Here's how the part is built. I have some questions about the finished solid (model axes, mm). A direction names the side the tool comes from. Give positions to 0.01 mm unless a question says otherwise; leave off trailing zeros. Order: outer loops, then holes, each group sorted by start corner. A loop starts at its lowest first (then second) coordinate and runs counter-clockwise, first axis right, second up. Notation, with made-up numbers: (21.5, 71.5) -> (32.5, 71.5) arc R20 cw to (32.5, 90.5) -> close; hole circle Ø10 at (-34, 8.25). An arc over 180 degrees is marked (long way). Write each question's results on one line, items separated by ' | '. Start each with the question number.
Q1. Imagine slicing it at D-D, the plane z = -16.5. Please give me the cut outline in (x, y), then the cut area to 3 significant figures.
Q2. Thinking about a two-plate mould opening in Z: for faces 1 (the face through (3.13, 28.27, -28.19)), 2 (the face through (3, 0, -26)), 3 (the face through (3.131, 1.528, -1.449)), which applies, pulls with the +Z half, pulls with the -Z half, needs draft (parallel to the pull), parting line crosses it, or undercut?
Q3. Imagine slicing it at A-A, the plane y = 51.5. Please give me the cut outline in (x, z).
Q4. Imagine slicing it at B-B, the plane z = -23. Please give me the cut outline in (x, y).
Q5. I need wall thicknesses on line 1 along Z through (x, y) = (4.75, 51); line 2 along Y through (x, z) = (5, -22); line 3 along Y through (x, z) = (1, -19). Which ranges of each line are inside material? Lowest first, please. Write a range as [from, to].
Q6. I'm going to push flat-ended pins straight in: pin 1 (1.9 mm diameter, centred on x = 4.5, y = 17.5, fed in from +Z); pin 2 (1.9 mm diameter, centred on x = 1.5, y = 2.5, fed in from +Z). Where does each tip first touch, or does it pass through?
Q7. For faces 4 (the face through (3, 29.718, -13)), 5 (the face through (3, 49, -29.718)), 6 (the face through (3, 33, -14.859)), which set-ups out of +Z, -Z, +X, -X, +Y, -Y let a thin tool reach every point of the face, with its end or its side?
Q8. Imagine slicing it at C-C, the plane x = 1. Please give me the cut outline in (y, z).
```python
from build123d import *

# Parameters (mm, degrees)
BOSS_EXTRUDE1_DEPTH = 6.35


with BuildPart() as part:
    # Sketch2 → Boss-Extrude1 (new body)
    with BuildSketch(Plane(origin=(0, 0, 0), x_dir=(0, 0, -1), z_dir=(1, 0, 0))):
        with BuildLine():
            Line((21.209, 0), (30.988, 0))
            ThreePointArc((30.988, 0), (34.580102448, 1.487897552), (36.068, 5.08))
            Line((36.068, 5.08), (36.068, 36.068))
            Line((36.068, 36.068), (36.068, 55.118))
            Line((36.068, 55.118), (29.718, 55.118))
            Line((29.718, 55.118), (29.718, 42.418))
            Line((29.718, 42.418), (6.35, 42.418))
            Line((6.35, 42.418), (6.35, 55.118))
            Line((6.35, 55.118), (0, 55.118))
            Line((0, 55.118), (0, 36.068))
            Line((0, 36.068), (0, 5.08))
            ThreePointArc((0, 5.08), (1.487897552, 1.487897552), (5.08, 0))
            Line((5.08, 0), (14.859, 0))
            Line((14.859, 0), (14.859, 6.35))
            Line((14.859, 6.35), (11.43, 6.35))
            ThreePointArc((11.43, 6.35), (7.837897552, 7.837897552), (6.35, 11.43))
            Line((6.35, 11.43), (6.35, 24.638))
            ThreePointArc((6.35, 24.638), (7.837897552, 28.230102448), (11.43, 29.718))
            Line((11.43, 29.718), (14.859, 29.718))
            Line((14.859, 29.718), (14.859, 36.068))
            Line((14.859, 36.068), (21.209, 36.068))
            Line((21.209, 36.068), (21.209, 29.718))
            Line((21.209, 29.718), (24.638, 29.718))
            ThreePointArc((24.638, 29.718), (28.230102448, 28.230102448), (29.718, 24.638))
            Line((29.718, 24.638), (29.718, 11.43))
            ThreePointArc((29.718, 11.43), (28.230102448, 7.837897552), (24.638, 6.35))
            Line((24.638, 6.35), (21.209, 6.35))
            Line((21.209, 6.35), (21.209, 0))
        make_face()
    extrude(amount=BOSS_EXTRUDE1_DEPTH)


solid = part.part
```
Geometry check:
1) outline: (0, 36.07) -> (6.35, 36.07) -> (6.35, 42.42) -> (0, 42.42) -> close | area: 40.3 mm²
2) face 1: undercut | face 2: needs draft | face 3: pulls with the +Z half
3) outline: (0, -36.07) -> (6.35, -36.07) -> (6.35, -29.72) -> (0, -29.72) -> close; (0, -6.35) -> (6.35, -6.35) -> (6.35, 0) -> (0, 0) -> close
4) outline: (0, 0) -> (6.35, 0) -> (6.35, 6.35) -> (0, 6.35) -> close; (0, 29.72) -> (6.35, 29.72) -> (6.35, 42.42) -> (0, 42.42) -> close
5) line 1: [-36.07, -29.72], [-6.35, 0] | line 2: [0, 6.35], [29.72, 42.42] | line 3: [36.07, 42.42]
6) pin 1: z = 0 | pin 2: z = -0.27
7) face 4: +X, -X | face 5: +X, -X, +Y | face 6: +X, -X, -Y
8) outline: (0, -30.99) arc R5.08 ccw to (5.08, -36.07) -> (55.12, -36.07) -> (55.12, -29.72) -> (42.42, -29.72) -> (42.42, -6.35) -> (55.12, -6.35) -> (55.12, 0) -> (5.08, 0) arc R5.08 ccw to (0, -5.08) -> (0, -14.86) -> (6.35, -14.86) -> (6.35, -11.43) arc R5.08 cw to (11.43, -6.35) -> (24.64, -6.35) arc R5.08 cw to (29.72, -11.43) -> (29.72, -14.86) -> (36.07, -14.86) -> (36.07, -21.21) -> (29.72, -21.21) -> (29.72, -24.64) arc R5.08 cw to (24.64, -29.72) -> (11.43, -29.72) arc R5.08 cw to (6.35, -24.64) -> (6.35, -21.21) -> (0, -21.21) -> close
